```python
from build123d import *

# Parameters (mm, degrees)
SKETCH1_R           = 8.89
BOSS_EXTRUDE1_DEPTH = 8.382
SKETCH15_W          = 3.175
SKETCH15_H          = 27.94
CUT_EXTRUDE14_DEPTH = 238.219932461
FILLET4_R           = 2.54


with BuildPart() as part:
    # Sketch1 → Boss-Extrude1 (new body)
    with BuildSketch(Plane(origin=(0, 0, 0), x_dir=(1, 0, 0), z_dir=(0, 1, 0))):
        with BuildLine():
            Line((-15.926997076, 224.074744797), (43.763002924, 224.074744797))
            ThreePointArc((43.763002924, 224.074744797), (46.457079761, 222.958821634), (47.573002924, 220.264744797))
            Line((47.573002924, 220.264744797), (47.573002924, 192.324744797))
            ThreePointArc((47.573002924, 192.324744797), (46.829054148, 190.528693573), (45.033002924, 189.784744797))
            Line((45.033002924, 189.784744797), (34.619002924, 189.784744797))
            ThreePointArc((34.619002924, 189.784744797), (32.8229517, 189.040796021), (32.079002924, 187.244744797))
            Line((32.079002924, 187.244744797), (32.079002924, 185.974744797))
            ThreePointArc((32.079002924, 185.974744797), (32.8229517, 184.178693573), (34.619002924, 183.434744797))
            Line((34.619002924, 183.434744797), (74.878002924, 183.434744797))
            ThreePointArc((74.878002924, 183.434744797), (76.674054148, 182.690796021), (77.418002924, 180.894744797))
            Line((77.418002924, 180.894744797), (77.418002924, -51.515255203))
            Line((77.418002924, -51.515255203), (52.526002924, -51.515255203))
            Line((52.526002924, -51.515255203), (49.667478553, -59.368986367))
            ThreePointArc((49.667478553, -59.368986367), (48.737543444, -60.580901395), (47.280659296, -61.040255203))
            Line((47.280659296, -61.040255203), (-19.444653447, -61.040255203))
            ThreePointArc((-19.444653447, -61.040255203), (-20.901537596, -60.580901395), (-21.831472704, -59.368986367))
            Line((-21.831472704, -59.368986367), (-24.689997076, -51.515255203))
            Line((-24.689997076, -51.515255203), (-49.581997076, -51.515255203))
            Line((-49.581997076, -51.515255203), (-49.581997076, 180.894744797))
            ThreePointArc((-49.581997076, 180.894744797), (-48.8380483, 182.690796021), (-47.041997076, 183.434744797))
            Line((-47.041997076, 183.434744797), (-6.782997076, 183.434744797))
            ThreePointArc((-6.782997076, 183.434744797), (-4.986945852, 184.178693573), (-4.242997076, 185.974744797))
            Line((-4.242997076, 185.974744797), (-4.242997076, 187.244744797))
            ThreePointArc((-4.242997076, 187.244744797), (-4.986945852, 189.040796021), (-6.782997076, 189.784744797))
            Line((-6.782997076, 189.784744797), (-17.196997076, 189.784744797))
            ThreePointArc((-17.196997076, 189.784744797), (-18.9930483, 190.528693573), (-19.736997076, 192.324744797))
            Line((-19.736997076, 192.324744797), (-19.736997076, 220.264744797))
            ThreePointArc((-19.736997076, 220.264744797), (-18.621073912, 222.958821634), (-15.926997076, 224.074744797))
        make_face()
        with Locations(Location((13.918002924, 206.294744797, 0), (0, 0, 270))):
            Circle(SKETCH1_R, mode=Mode.SUBTRACT)
    extrude(amount=BOSS_EXTRUDE1_DEPTH)

    # Sketch15 → Cut-Extrude14 (cut, through all)
    with BuildSketch(Plane(origin=(0, 8.382, 0), x_dir=(-1, 0, 0), z_dir=(0, 1, 0))):
        with Locations((47.994497076, -169.464744797)):
            Rectangle(SKETCH15_W, SKETCH15_H)
        with Locations((-75.830502924, -169.464744797)):
            Rectangle(SKETCH15_W, SKETCH15_H)
    extrude(amount=-CUT_EXTRUDE14_DEPTH, mode=Mode.SUBTRACT)

    # Fillet4
    fillet4_edges = [part.edges().sort_by_distance(p)[0] for p in [
        (74.243002924, 4.191, -183.434744797),
        (77.418002924, 4.191, -155.494744797),
        (-49.581997076, 4.191, 51.515255203),
        (77.418002924, 4.191, 51.515255203),
        (-49.581997076, 4.191, -155.494744797),
        (-46.406997076, 4.191, -183.434744797),
    ]]
    fillet(fillet4_edges, radius=FILLET4_R)


solid = part.part
```
Model file for the job. Use its own axes, mm. A direction names the side the tool comes from. Give positions to 0.01 mm unless a question says otherwise; leave off trailing zeros. Order: outer loops, then holes, each group sorted by start corner. A loop starts at its lowest first (then second) coordinate and runs counter-clockwise, first axis right, second up.
1) Saw through at A-A, the plane x = -33. Write the cut outline in (y, z), then the cut area to 3 significant figures.
2) Mould opens along Z. For faces 4 (the flat face through (-12, 4, -189.785)), 5 (the flat face through (-46.407, 4, -168)), 6 (the flat face through (-36, 4, 51.515)) say: +Z half, -Z half, draft (parallel to the pull), parting line (faces both ways), or undercut.
3) Wall check: probe 1 along Z at (x, y) = (35, 7); probe 2 along Z at (x, y) = (58, 1); probe 3 along Z at (x, y) = (20.5, 2.75). Give the ranges that are in metal, low to high.
4) 3-axis set-ups, long thin cutter, end or side, ignore diameter. For faces 1 (the flat face through (-26, 4, -183.435)), 2 (the flat face through (-19.737, 4, -206)), 3 (the flat face through (53, 4, -183.435)): which of +Z, -Z, +X, -X, +Y, -Y reach the whole face in a straight line?
5) Pin check, flat tips, straight feed: pin 1 (4 mm diameter, centred on y = 2.5, z = -203.5, fed in from -X); pin 2 (23 mm diameter, centred on x = 13.92, z = -206.29, fed in from +Y); pin 3 (1.4 mm diameter, centred on y = 2.5, z = -186.5, fed in from +X) (3 decimals); pin 4 (4 mm diameter, centred on x = -21, y = 4, fed in from -Z). Stop position of each tip, or through.
Computed:
1. outline: (0, -183.43) - (8.38, -183.43) - (8.38, 51.52) - (0, 51.52) - close
1. area: 1,970 mm2
2. face 4: undercut
2. face 5: draft
2. face 6: +Z half
3. probe 1: z = -224.07 to -189.78, -183.43 to 61.04
3. probe 2: z = -183.43 to 51.52
3. probe 3: z = -224.07 to -212.27, -200.32 to 61.04
4. face 1: -X, +Y, -Y
4. face 2: -Z, -X, +Y, -Y
4. face 3: +X, +Y, -Y
5. pin 1: stops at x = -19.74
5. pin 2: stops at y = 8.38
5. pin 3: stops at x = 32.085
5. pin 4: stops at z = -222.52
